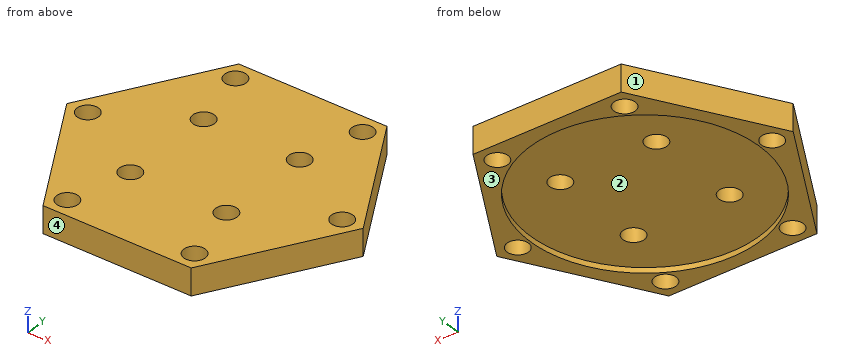
```python
from build123d import *

# Parameters (mm, degrees)
EXTRUDE_1_DEPTH     = 5
SKETCH_11_R         = 21.35
CUT_EXTRUDE_1_DEPTH = 1
F_4_0MM_2_D         = 4
F_4_0MM_3_OUTLINE_R = 2
F_4_0MM_3_DEPTH     = 5


# Read off the part's stored shape, not the designer's step: Ø4.0mm 暗销孔3
with BuildPart() as part:
    # 草图2 → 凸台-拉伸1 (new body)
    with BuildSketch(Plane.XY):
        Polygon((-13.856406461, 24), (-27.712812921, 0), (-13.856406461, -24), (13.856406461, -24), (27.712812921, 0), (13.856406461, 24), align=None)
    extrude(amount=EXTRUDE_1_DEPTH)

    # 草图11 → 切除-拉伸1 (cut)
    with BuildSketch(Plane(origin=(0, 0, 0), x_dir=(-1, 0, 0), z_dir=(0, 0, -1))):
        Circle(SKETCH_11_R)
    extrude(amount=-CUT_EXTRUDE_1_DEPTH, mode=Mode.SUBTRACT)

    # Ø4.0mm 暗销孔2 (through all)
    with Locations(Plane(origin=(0, 0, 1), x_dir=(-1, 0, 0), z_dir=(0, 0, -1))):
        with Locations((8.980256121, 8.980256121), (-8.980256121, 8.980256121), (-8.980256121, -8.980256121), (8.980256121, -8.980256121)):
            Hole(F_4_0MM_2_D / 2)

    # Ø4.0mm 暗销孔3 outline → Ø4.0mm 暗销孔3 (cut)
    with BuildSketch(Plane.XY):
        with Locations((23.786831091, 0)):
            Circle(F_4_0MM_3_OUTLINE_R)
        with Locations((-11.893415545, -20.6)):
            Circle(F_4_0MM_3_OUTLINE_R)
        with Locations((11.893415545, -20.6)):
            Circle(F_4_0MM_3_OUTLINE_R)
        with Locations((-23.786831091, 0)):
            Circle(F_4_0MM_3_OUTLINE_R)
        with Locations((-11.893415545, 20.6)):
            Circle(F_4_0MM_3_OUTLINE_R)
        with Locations((11.893415545, 20.6)):
            Circle(F_4_0MM_3_OUTLINE_R)
    extrude(amount=F_4_0MM_3_DEPTH, mode=Mode.SUBTRACT)


solid = part.part
```
Geometry: final body of the model. Coordinates: model frame, mm. Face numbers are marked on the shaded views. Round coordinates to 2 decimals unless told otherwise and drop trailing zeros. Order: outer loops, then holes, each group sorted by start corner. A loop starts at its lowest first (then second) coordinate and runs counter-clockwise, first axis right, second up. Notation, with made-up numbers: (70, -11.75) - (100, -11.75) arc R32 ccw to (100, 14.25) - close; hole circle Ø9 at (-13.75, 20.5). An arc over 180 degrees is marked (long way). Write item = value, one per line. Start each with the question number.
Q1. Cut plane A-A on y = -8. Return the cut outline in (x, z).
Q2. Cut plane C-C on z = 2.7. Give the number of separate pieces and of enclosed holes in the cut face, and give its area (3 significant figures).
Q3. Pin query (flat end, axial travel): pin 1 (4 mm diameter, centred on x = -15, y = -5, fed in from -Z); pin 2 (1.5 mm diameter, centred on y = 18, z = 4.5, fed in from +X). Return the tip coordinate at first contact, or that it passes through.
Q4. Cut plane D-D on x = 8. Return the cut outline in (y, z).
Q5. Ray query, line 1 (Y direction, x = -9, z = 3.65); line 2 (Z direction, x = 0, y = 14.5); line 3 (Y direction, x = -13, z = 1.85). Return the intervals inside material, ascending. Write a range as from..to.
Q6. Pull-direction query (Y, two-part tool) for the marked faces 1, 2, 3 and 4; classes: +Y half, -Y half, draft (parallel to the pull), parting line (faces both ways), or undercut.
Q7. Cut plane B-B on x = 0. Return the cut outline in (y, z), and give its area (3 significant figures).
Outcome:
q1.outline = (-23.09, 0) - (-19.79, 0) - (-19.79, 1) - (-10.72, 1) - (-10.72, 5) - (-23.09, 5) - close; (-7.24, 1) - (7.24, 1) - (7.24, 5) - (-7.24, 5) - close; (10.72, 1) - (19.79, 1) - (19.79, 0) - (23.09, 0) - (23.09, 5) - (10.72, 5) - close
q2.separate_pieces = 1
q2.enclosed_holes = 10
q2.area = 1,870 mm^2
q3.pin_1 = 1
q3.pin_2 = 17.75
q4.outline = (-24, 0) - (-19.79, 0) - (-19.79, 1) - (-10.72, 1) - (-10.72, 5) - (-24, 5) - close; (-7.24, 1) - (7.24, 1) - (7.24, 5) - (-7.24, 5) - close; (10.72, 1) - (19.79, 1) - (19.79, 0) - (24, 0) - (24, 5) - (10.72, 5) - close
q5.line_1 = -24..-10.98, -6.98..6.98, 10.98..24
q5.line_2 = 1..5
q5.line_3 = -24..-22.27, -18.93..18.93, 22.27..24
q6.face_1 = +Y half
q6.face_2 = undercut
q6.face_3 = draft
q6.face_4 = -Y half
q7.outline = (-24, 0) - (-21.35, 0) - (-21.35, 1) - (21.35, 1) - (21.35, 0) - (24, 0) - (24, 5) - (-24, 5) - close
q7.area = 197 mm^2
